```python
from build123d import *

# Parameters (mm, degrees)
SKETCH001_W  = 249.235731
SKETCH001_H  = 289.366922
PAD_DEPTH    = 4
PAD001_DEPTH = 93
PAD002_DEPTH = 36


with BuildPart() as part:
    # Sketch001 → Pad (new body)
    with BuildSketch(Plane.XY):
        with Locations((101.953362, -122.984355)):
            Rectangle(SKETCH001_W, SKETCH001_H)
    extrude(amount=PAD_DEPTH)

    # Sketch (on Face6 of Pad) → Pad001 (join)
    with BuildSketch(Plane.XY.offset(4)):
        Polygon((-17, -135.5), (0, -135.5), (0, -106), (-5, -106), (-5, -130.5), (-22, -130.5), (-22, -263.55), (-17, -263.55), align=None)
        Polygon((0, 0), (32, 0), (32, 5), (-5, 5), (-5, -73), (0, -73), align=None)
        Polygon((66, 5), (66, 0), (190, 0), (211.023543, -21.401183), (211.023543, -89.401183), (189.213253, -110), (138.213253, -110), (138.213253, -125), (143.213253, -125), (143.213253, -115), (191.201161, -115), (216.023543, -91.5564), (216.023543, -19.356138), (192.097187, 5), align=None)
        Polygon((138.2, -257.999998), (28.2, -257.999998), (28.2, -221.999998), (23.2, -221.999998), (23.2, -262.999998), (143.2, -262.999998), (143.2, -174.999998), (138.2, -174.999998), align=None)
    extrude(amount=PAD001_DEPTH)

    # Sketch002 (on Face5 of Pad001) → Pad002 (join)
    with BuildSketch(Plane.XY.offset(4)):
        Polygon((138.213253, -116), (43.213253, -116), (43.213253, -154), (94.889137, -154), (112.213253, -171.324116), (112.213253, -232.1), (65.2, -232.1), (65.2, -258.1), (138.213253, -258.1), align=None)
    extrude(amount=PAD002_DEPTH)


solid = part.part
```
Design review of the part built by this model. Coordinates are the model's own, in mm. A direction names the side the tool comes from. Round coordinates to 2 decimals unless told otherwise and drop trailing zeros. Write each loop counter-clockwise with the first axis right and the second up, starting at its lowest first coordinate (ties: lowest second). Pieces come first, ordered by that corner, then holes. Notation, with made-up numbers: (-21.75, -34) -> (15.25, -34) arc R31 ccw to (15.25, -9) -> close; hole circle Ø10 at (74.25, 86). An arc over 180 degrees is marked (long way). Answer in a Markdown table with one row per item.
Q1. Draft analysis for pull direction X (two halves, no side actions). For faces 1 (the face through (-13, -130.5, 50)), 2 (the face through (203.44, -103.44, 49.85)), 3 (the face through (211.024, -55, 50)), state which applies: +X half, -X half, draft (parallel to the pull), parting line (faces both ways), or undercut.
The answers:
| item | result |
|---|---|
| face 1 | draft |
| face 2 | +X half |
| face 3 | undercut |
Q2. Take a section at C-C, the plane z = 13. Count the separate pieces of the cut face and the enclosed holes in it, then the cut area to 3 significant figures.
The answers:
| item | result |
|---|---|
| separate pieces | 3 |
| enclosed holes | 0 |
| area | 11,900 mm² |
Q3. Take a section at B-B, the plane y = -247.5. State the section outline as (x, z) points.
The answers:
| item | result |
|---|---|
| outline | (-22.66, 0) -> (226.57, 0) -> (226.57, 4) -> (143.2, 4) -> (143.2, 97) -> (138.2, 97) -> (138.2, 40) -> (65.2, 40) -> (65.2, 4) -> (28.2, 4) -> (28.2, 97) -> (23.2, 97) -> (23.2, 4) -> (-17, 4) -> (-17, 97) -> (-22, 97) -> (-22, 4) -> (-22.66, 4) -> close |
Q4. Clearance check with flat-ended pins moving along their axes: pin 1 Ø3 at (x, z) = (164.5, 57.5) entering from -Y; pin 2 Ø4 at (x, z) = (141.5, 49.5) entering from +Y; pin 3 Ø1.5 at (x, z) = (46.5, 12) entering from -Y; pin 4 Ø5 at (x, y) = (37, -71.5) entering from -Z. State where each tip first meets the part, or that it passes through.
The answers:
| item | result |
|---|---|
| pin 1 | y = -115 |
| pin 2 | y = 5 |
| pin 3 | y = -263 |
| pin 4 | z = 0 |
Q5. Take a section at D-D, the plane y = -199. State the section outline as (x, z) points, then the cut area to 3 significant figures.
The answers:
| item | result |
|---|---|
| outline | (-22.66, 0) -> (226.57, 0) -> (226.57, 4) -> (143.2, 4) -> (143.2, 97) -> (138.2, 97) -> (138.2, 40) -> (112.21, 40) -> (112.21, 4) -> (-17, 4) -> (-17, 97) -> (-22, 97) -> (-22, 4) -> (-22.66, 4) -> close |
| area | 2,860 mm² |
Q6. Take a section at A-A, the plane x = 126. State the section outline as (y, z) points.
The answers:
| item | result |
|---|---|
| outline | (-267.67, 0) -> (21.7, 0) -> (21.7, 4) -> (5, 4) -> (5, 97) -> (0, 97) -> (0, 4) -> (-116, 4) -> (-116, 40) -> (-258, 40) -> (-258, 97) -> (-263, 97) -> (-263, 4) -> (-267.67, 4) -> close |
Q7. For faces 4 (the face through (143.2, -220, 50)), 5 (the face through (69, -154, 22)), 6 (the face through (14, 5, 50)), 7 (the face through (-5, -33, 50)), 8 (the face through (-9, -135.5, 50)), list the 3-axis set-ups (+Z, -Z, +X, -X, +Y, -Y) from which the entire face can be reached by the end or side of a thin tool; tool diameter is ignored.
The answers:
| item | result |
|---|---|
| face 4 | +Z, +X, -Y |
| face 5 | +Z |
| face 6 | +Z, +X, -X, +Y |
| face 7 | +Z, -X, +Y |
| face 8 | +Z, -Y |
Q8. To check wall thickness, follow L1, parallel to X at y = -60.5, z = 34; L2, parallel to Y at x = 57, z = 7; L3, parallel to Y at x = 105, z = 9.5. State the ranges of each line that lie inside material, in increasing order. Write a range as [from, to].
The answers:
| item | result |
|---|---|
| L1 | [-5, 0], [211.02, 216.02] |
| L2 | [-263, -258], [-154, -116] |
| L3 | [-263, -232.1], [-164.11, -116], [0, 5] |
